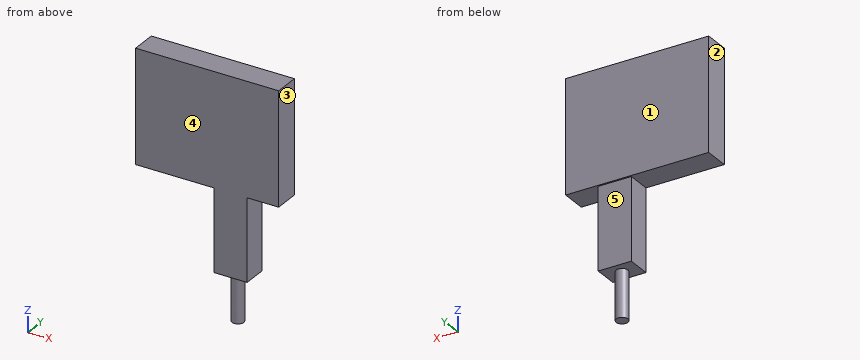
```python
from build123d import *

# Parameters (mm, degrees)
SKETCH1_W           = 90.6
SKETCH1_H           = 71.5
BOSS_EXTRUDE1_DEPTH = 16
SKETCH2_W           = 21
SKETCH2_H           = 52
BOSS_EXTRUDE2_DEPTH = 15
SKETCH3_R           = 3.75
BOSS_EXTRUDE3_DEPTH = 30


with BuildPart() as part:
    # Sketch1 → Boss-Extrude1 (new body)
    with BuildSketch(Plane(origin=(0, 0, 0), x_dir=(1, 0, 0), z_dir=(0, 1, 0))):
        Rectangle(SKETCH1_W, SKETCH1_H)
    extrude(amount=BOSS_EXTRUDE1_DEPTH)

    # Sketch2 → Boss-Extrude2 (add)
    with BuildSketch(Plane(origin=(0, 0, 0), x_dir=(1, 0, 0), z_dir=(0, 1, 0))):
        with Locations((14.8, 61.75)):
            Rectangle(SKETCH2_W, SKETCH2_H)
    extrude(amount=BOSS_EXTRUDE2_DEPTH)

    # Sketch3 → Boss-Extrude3 (add)
    with BuildSketch(Plane(origin=(0, 0, -87.75), x_dir=(-1, 0, 0), z_dir=(0, 0, -1))):
        with Locations((-14.8, 7.5)):
            Circle(SKETCH3_R)
    extrude(amount=BOSS_EXTRUDE3_DEPTH)


solid = part.part
```
Geometry check sheet. Reference: the model listing, model coordinates, mm. Face numbers are marked on the shaded views. A direction names the side the tool comes from. Give positions to 0.01 mm unless a question says otherwise; leave off trailing zeros. Order: outer loops, then holes, each group sorted by start corner. A loop starts at its lowest first (then second) coordinate and runs counter-clockwise, first axis right, second up. Notation, with made-up numbers: (39.5, -6.5) - (87.5, -6.5) arc R18 ccw to (87.5, 10.5) - close; hole circle Ø10 at (36.5, 2.5). An arc over 180 degrees is marked (long way). Answer in a Markdown table with one row per item. Add a question column.
Q1. Cross-section at A-A, the plane y = 2.25. Enter the section's corners in (x, z).
Q2. Cross-section at D-D, the plane x = -19. Enter the section's corners in (y, z), then the cut area to 3 significant figures.
Q3. Mould release check, pull along X, two halves, no side actions. Record for the marked faces 1, 2 and 3: pulls with the +X half, pulls with the -X half, needs draft (parallel to the pull), parting line crosses it, or undercut.
Q4. Cross-section at B-B, the plane x = 14.8. Enter the section's corners in (y, z), then the cut area to 3 significant figures.
Q5. Cross-section at C-C, the plane z = -39.5. Enter the section's corners in (x, y).
Q6. Gauge pin test, flat ends, axial feed: pin 1 (4 mm diameter, centred on y = 9, z = -76.5, fed in from +X); pin 2 (23 mm diameter, centred on x = 13, z = -52, fed in from +Y); pin 3 (12 mm diameter, centred on x = -4, z = -85.5, fed in from +Y); pin 4 (6 mm diameter, centred on x = 0.5, y = 14, fed in from -Z). Record the tip position at first contact, or that the pin passes through.
Q7. Material ranges on probe 1 along Z at (x, y) = (11.5, 5.25); probe 2 along Z at (x, y) = (-40.5, 3); probe 3 along X at (y, z) = (8, -80), recorded low to high. Write a range as from..to.
Q8. Tool access check on the marked faces 4 and 5. Record the directions out of +Z, -Z, +X, -X, +Y, -Y that give a thin tool (end or side, any length) a straight path to the whole face; none if there is none.
Check values:
| question | item | result |
|---|---|---|
| 1 | outline | (-45.3, -35.75) - (4.3, -35.75) - (4.3, -87.75) - (25.3, -87.75) - (25.3, -35.75) - (45.3, -35.75) - (45.3, 35.75) - (-45.3, 35.75) - close |
| 2 | outline | (0, -35.75) - (16, -35.75) - (16, 35.75) - (0, 35.75) - close |
| 2 | area | 1,140 mm^2 |
| 3 | face 1 | needs draft |
| 3 | face 2 | pulls with the -X half |
| 3 | face 3 | pulls with the +X half |
| 4 | outline | (0, -87.75) - (3.75, -87.75) - (3.75, -117.75) - (11.25, -117.75) - (11.25, -87.75) - (15, -87.75) - (15, -35.75) - (16, -35.75) - (16, 35.75) - (0, 35.75) - close |
| 4 | area | 2,150 mm^2 |
| 5 | outline | (4.3, 0) - (25.3, 0) - (25.3, 15) - (4.3, 15) - close |
| 6 | pin 1 | stops at x = 25.3 |
| 6 | pin 2 | stops at y = 15 |
| 6 | pin 3 | passes through |
| 6 | pin 4 | stops at z = -35.75 |
| 7 | probe 1 | z = -87.75..35.75 |
| 7 | probe 2 | z = -35.75..35.75 |
| 7 | probe 3 | x = 4.3..25.3 |
| 8 | face 4 | +Z, -Z, +X, -X, -Y |
| 8 | face 5 | -Z, +X, -X, +Y |
